Could you check a few things on this model? Use its own coordinates, in mm. A direction names the side the tool comes from. Give positions to 0.01 mm unless a question says otherwise; leave off trailing zeros. Loops run counter-clockwise (first coordinate to the right, second up) from the corner with the lowest first, then second, coordinate; pieces in that order, holes last. Notation, with made-up numbers: (58.5, 49) -> (84.5, 49) arc R24 cw to (84.5, 59) -> close; hole circle Ø1 at (-31.5, -16). An arc over 180 degrees is marked (long way). Write each question's results on one line, items separated by ' | '. Start each with the question number.
Q1. We'd pull the mould along Y, two halves only. Please class faces 5 (the face through (-97.461, 143, 299)), 6 (the face through (0, -2, 226)), 7 (the face through (-63, 2, 361.95)), 8 (the face through (-27, 152.4, 232)): released by +Y, released by -Y, zero draft, split by the parting line, or undercut.
Q2. If we section it at A-A, the plane y = 103: List the corners of the cut face in (x, z) for me, plus the area to 3 significant figures.
Q3. If we section it at D-D, the plane x = 72: List the corners of the cut face in (y, z) for me.
Q4. If we section it at B-B, the plane z = 314: List the corners of the cut face in (x, y) for me.
Q5. Will these pins go through, and if not, where does the flat tip stop? P1, Ø21, axis at x = -35.5, y = 139.5, coming from the -Z side; P2, Ø5.5, axis at y = -17.5, z = 221, coming from the -X side; P3, Ø8, axis at x = -97, y = 1, coming from the +Z side.
Q6. If we section it at C-C, the plane x = -59: List the corners of the cut face in (y, z) for me.
Q7. If I drill on line 1 along Y through (x, z) = (28, 318.5); line 2 along Z through (x, y) = (-89, 120.5); line 3 along X through (y, z) = (123, 362), over which ranges is the centre line in solid material (lowest first)?
Q8. Which directions (+Z, -Z, +X, -X, +Y, -Y) give clear straight access to the entire face, cutting with the end or side of a thin tool? Please do faces 1 (the face through (92.974, 143.008, 102.814)), 2 (the face through (-6.8, -143, 308.6)), 3 (the face through (-7.016, -143.008, 453.044)), 4 (the face through (-27, -133.35, 224)).
from build123d import *

# Parameters (mm, degrees)
F5_DEPTH  = 19.05
F6_DEPTH  = 19.05
F7_W      = 279.4
F7_H      = 19.05
F8_DEPTH  = 112.776
F9_W      = 279.4
F9_H      = 19.05
F10_DEPTH = 209.804
F12_DEPTH = 375.92
F15_DEPTH = 313.436


with BuildPart() as f5:
    # F4 (on offset) → F5 (new body)
    with BuildSketch(Plane.XZ.offset(152.4)):
        with BuildLine():
            Line((156.056568, 0), (163.756519, 0))
            ThreePointArc((163.756519, 0), (185.111738, 11.648106), (186.880512, 35.909087))
            Line((186.880512, 35.909087), (2.185208, 442.309087))
            ThreePointArc((2.185208, 442.309087), (-7.186892, 453.15522), (-20.938786, 457.2))
            Line((-20.938786, 457.2), (-135.561358, 457.2))
            ThreePointArc((-135.561358, 457.2), (-153.52187, 449.760512), (-160.961358, 431.8))
            Line((-160.961358, 431.8), (-160.961358, 25.4))
            ThreePointArc((-160.961358, 25.4), (-153.52187, 7.439488), (-135.561358, 0))
            Line((-135.561358, 0), (-122.861358, 0))
            ThreePointArc((-122.861358, 0), (-104.900846, 7.439488), (-97.461358, 25.4))
            Line((-97.461358, 25.4), (-97.461358, 177.8))
            ThreePointArc((-97.461358, 177.8), (-90.02187, 195.760512), (-72.061358, 203.2))
            Line((-72.061358, 203.2), (30.995779, 203.2))
            ThreePointArc((30.995779, 203.2), (44.747674, 199.15522), (54.119773, 188.309087))
            Line((54.119773, 188.309087), (132.932575, 14.890913))
            ThreePointArc((132.932575, 14.890913), (142.304674, 4.04478), (156.056568, 0))
        make_face()
    extrude(amount=-F5_DEPTH)



with BuildPart() as f6:
    # F3 (on offset) → F6 (new body)
    with BuildSketch(Plane.XZ.offset(-152.4)):
        with BuildLine():
            Line((156.056568, 0), (163.756519, 0))
            ThreePointArc((163.756519, 0), (185.111738, 11.648106), (186.880512, 35.909087))
            Line((186.880512, 35.909087), (2.185208, 442.309087))
            ThreePointArc((2.185208, 442.309087), (-7.186892, 453.15522), (-20.938786, 457.2))
            Line((-20.938786, 457.2), (-135.561358, 457.2))
            ThreePointArc((-135.561358, 457.2), (-153.52187, 449.760512), (-160.961358, 431.8))
            Line((-160.961358, 431.8), (-160.961358, 25.4))
            ThreePointArc((-160.961358, 25.4), (-153.52187, 7.439488), (-135.561358, 0))
            Line((-135.561358, 0), (-122.861358, 0))
            ThreePointArc((-122.861358, 0), (-104.900846, 7.439488), (-97.461358, 25.4))
            Line((-97.461358, 25.4), (-97.461358, 177.8))
            ThreePointArc((-97.461358, 177.8), (-90.02187, 195.760512), (-72.061358, 203.2))
            Line((-72.061358, 203.2), (30.995779, 203.2))
            ThreePointArc((30.995779, 203.2), (44.747674, 199.15522), (54.119773, 188.309087))
            Line((54.119773, 188.309087), (132.932575, 14.890913))
            ThreePointArc((132.932575, 14.890913), (142.304674, 4.04478), (156.056568, 0))
        make_face()
    extrude(amount=F6_DEPTH)


with BuildPart() as f5_1:
    add(f5.part)

    add(f6.part)  # F8 merges F6
    # F7 (on Right) → F8 (join)
    with BuildSketch(Plane.YZ):
        with Locations((0, 225.425)):
            Rectangle(F7_W, F7_H)
    extrude(amount=F8_DEPTH)

    # F9 (on face) → F10 (join)
    with BuildSketch(Plane(origin=(-160.961358, 0, 0), x_dir=(0, -1, 0), z_dir=(-1, 0, 0))):
        with Locations((0, 371.475)):
            Rectangle(F9_W, F9_H)
    extrude(amount=-F10_DEPTH)

    # F11 (on face) → F12 (cut)
    with BuildSketch(Plane(origin=(0, 152.4, 0), x_dir=(-1, 0, 0), z_dir=(0, 1, 0))):
        Polygon((-117.13268, 189.380877), (-14.780929, 414.593705), (-39.657071, 420.538783), (-147.453333, 203.160607), align=None)
    extrude(amount=-F12_DEPTH, mode=Mode.SUBTRACT)

    # F14 (on face) → F15 (cut)
    with BuildSketch(Plane.XZ.offset(152.4)):
        with BuildLine():
            ThreePointArc((-18.542245, 247.65), (2.812975, 259.298106), (4.581749, 283.559087))
            Line((4.581749, 283.559087), (-18.505164, 334.359087))
            ThreePointArc((-18.505164, 334.359087), (-27.877264, 345.20522), (-41.629158, 349.25))
            Line((-41.629158, 349.25), (-72.061358, 349.25))
            ThreePointArc((-72.061358, 349.25), (-90.02187, 341.810512), (-97.461358, 323.85))
            Line((-97.461358, 323.85), (-97.461358, 273.05))
            ThreePointArc((-97.461358, 273.05), (-90.02187, 255.089488), (-72.061358, 247.65))
            Line((-72.061358, 247.65), (-18.542245, 247.65))
        make_face()
    extrude(amount=-F15_DEPTH, mode=Mode.SUBTRACT)


solid = f5_1.part
Final values:
1) face 5: zero draft | face 6: undercut | face 7: undercut | face 8: released by +Y
2) outline: (-160.96, 361.95) -> (38.71, 361.95) -> (30.05, 381) -> (-160.96, 381) -> close; (0, 215.9) -> (105.08, 215.9) -> (96.42, 234.95) -> (0, 234.95) -> close | area: 5,640 mm²
3) outline: (-152.4, 148.97) -> (-133.35, 148.97) -> (-133.35, 215.9) -> (133.35, 215.9) -> (133.35, 148.97) -> (152.4, 148.97) -> (152.4, 288.69) -> (133.35, 288.69) -> (133.35, 234.95) -> (-133.35, 234.95) -> (-133.35, 288.69) -> (-152.4, 288.69) -> close
4) outline: (-160.96, -152.4) -> (-97.46, -152.4) -> (-97.46, -133.35) -> (-160.96, -133.35) -> close; (-160.96, 133.35) -> (-97.46, 133.35) -> (-97.46, 152.4) -> (-160.96, 152.4) -> close; (-9.25, -152.4) -> (60.5, -152.4) -> (60.5, -133.35) -> (-9.25, -133.35) -> close; (-9.25, 133.35) -> (60.5, 133.35) -> (60.5, 152.4) -> (-9.25, 152.4) -> close
5) P1: stops at z = 203.2 | P2: stops at x = 0 | P3: stops at z = 381
6) outline: (-152.4, 203.2) -> (-133.35, 203.2) -> (-133.35, 247.65) -> (-152.4, 247.65) -> close; (-152.4, 349.25) -> (-133.35, 349.25) -> (-133.35, 361.95) -> (133.35, 361.95) -> (133.35, 349.25) -> (152.4, 349.25) -> (152.4, 457.2) -> (133.35, 457.2) -> (133.35, 381) -> (-133.35, 381) -> (-133.35, 457.2) -> (-152.4, 457.2) -> close; (133.35, 203.2) -> (152.4, 203.2) -> (152.4, 247.65) -> (133.35, 247.65) -> close
7) line 1: y = -152.4 to -133.35, 133.35 to 152.4 | line 2: z = 361.95 to 381 | line 3: x = -160.96 to 38.68
8) face 1: -Z, +Y, -Y | face 2: +Y, -Y | face 3: +Z, +X, +Y, -Y | face 4: -X
